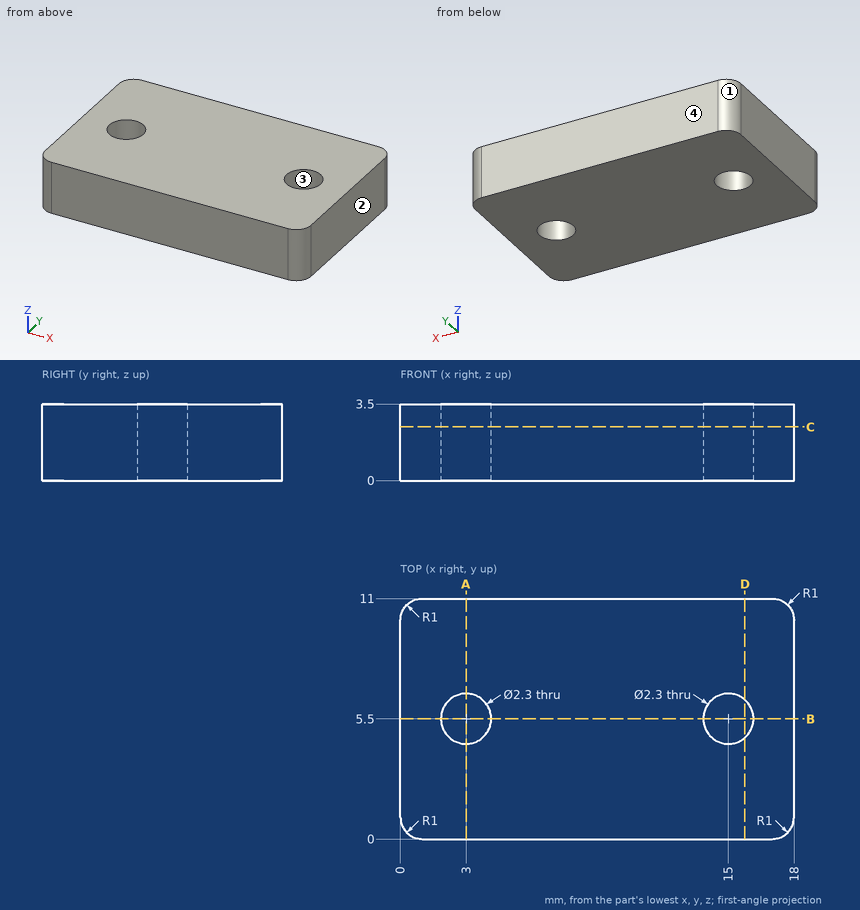
Study the drawing (mm; zero at the part's minimum x, y, z) and answer. Round coordinates to 2 decimals unless told otherwise and drop trailing zeros. Loops run counter-clockwise (first coordinate to the right, second up) from the corner with the lowest first, then second, coordinate; pieces in that order, holes last. Notation, with made-up numbers: (-2.75, 36) -> (42.25, 36) arc R19 ccw to (42.25, 41) -> close; hole circle Ø6 at (41, -38). An arc over 180 degrees is marked (long way). Use one line per item in the form item = value.
1. The part is cut by section D-D on x = 15.75. Determine the outline of the cut face in (y, z).
Answer key:
outline = (0, 0) -> (4.63, 0) -> (4.63, 3.5) -> (0, 3.5) -> close; (6.37, 0) -> (11, 0) -> (11, 3.5) -> (6.37, 3.5) -> close
2. The part is cut by section C-C on z = 2.45. Determine the outline of the cut face in (x, y).
Answer key:
outline = (0, 1) arc R1 ccw to (1, 0) -> (17, 0) arc R1 ccw to (18, 1) -> (18, 10) arc R1 ccw to (17, 11) -> (1, 11) arc R1 ccw to (0, 10) -> close; hole circle Ø2.3 at (3, 5.5); hole circle Ø2.3 at (15, 5.5)
3. The part is cut by section B-B on y = 5.5. Determine the outline of the cut face in (x, z).
Answer key:
outline = (0, 0) -> (1.85, 0) -> (1.85, 3.5) -> (0, 3.5) -> close; (4.15, 0) -> (13.85, 0) -> (13.85, 3.5) -> (4.15, 3.5) -> close; (16.15, 0) -> (18, 0) -> (18, 3.5) -> (16.15, 3.5) -> close
4. Find the intervals of material crossed by probe 1 along Y at (x, z) = (3, 2.65); probe 2 along X at (y, z) = (6, 2.9); probe 3 along X at (y, z) = (6.5, 0.85), in increasing order. Write a range as [from, to].
Answer key:
probe_1 = [0, 4.35], [6.65, 11]
probe_2 = [0, 1.96], [4.04, 13.96], [16.04, 18]
probe_3 = [0, 2.43], [3.57, 14.43], [15.57, 18]
5. For a pull along X with two mould halves and no side action, classify the marked faces 1, 2, 3 and 4 as released by +X, released by -X, zero draft, split by the parting line, or undercut.
Answer key:
face_1 = released by -X
face_2 = released by +X
face_3 = undercut
face_4 = zero draft
6. The part is cut by section A-A on x = 3. Determine the outline of the cut face in (y, z).
Answer key:
outline = (0, 0) -> (4.35, 0) -> (4.35, 3.5) -> (0, 3.5) -> close; (6.65, 0) -> (11, 0) -> (11, 3.5) -> (6.65, 3.5) -> close
